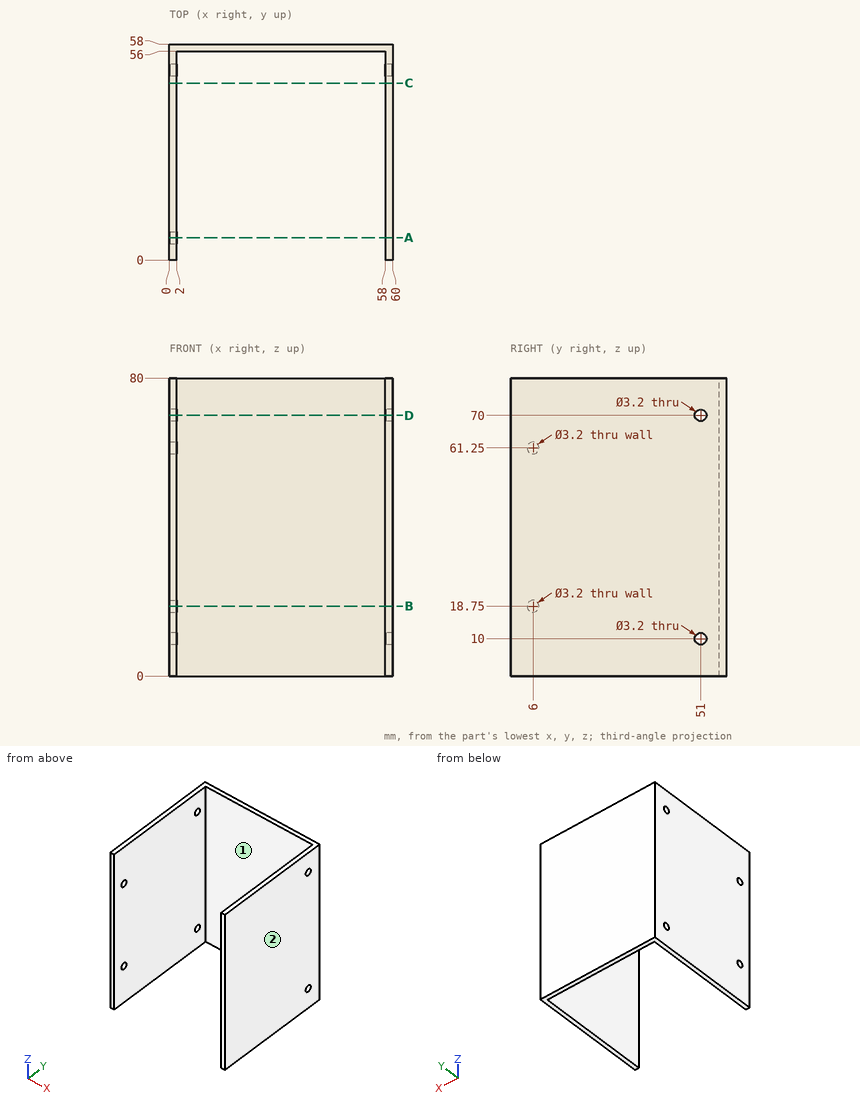
Part print with two shaded views. Sizes in mm from the minimum x, y, z corner. A direction names the side the tool comes from. Round coordinates to 2 decimals unless told otherwise and drop trailing zeros. Write each loop counter-clockwise with the first axis right and the second up, starting at its lowest first coordinate (ties: lowest second). Pieces come first, ordered by that corner, then holes. Notation, with made-up numbers: M 80,34.25 L 116,34.25 A24 ccw 116,58.25 Z; hole C -40,75.25 d4. An arc over 180 degrees is marked long. Answer as CSV lines item,"result". Start each with the question number.
1) Band-saw the part on A-A (y = 6). List the corners of the cut face in (x, z).
2) Band-saw the part on C-C (y = 47.5). List the corners of the cut face in (x, z), then the cut area to 3 significant figures.
3) Band-saw the part on D-D (z = 70). List the corners of the cut face in (x, y), then the cut area to 3 significant figures.
4) Band-saw the part on B-B (z = 18.75). List the corners of the cut face in (x, y).
5) Which spindle directions (+Z, -Z, +X, -X, +Y, -Y) get a long thin tool onto all of the face, cutting with end or side? Do the marked faces 1 and 2. Say none if no direction does.
6) Drill centre lines: L1, parallel to Z at x = 59, y = 51; L2, parallel to X at y = 25.5, z = 7; L3, parallel to Y at x = 0.65, z = 61.25. Where is each one in solid material? Low to high.
7) Drop flat-ended pins along their axis: pin 1 (1.9 mm diameter, centred on y = 51, z = 10, fed in from +X); pin 2 (3 mm diameter, centred on y = 6, z = 18.75, fed in from -X). Give the stop position or say it passes through.
Worked out:
1,outline,"M 0,0 L 2,0 L 2,17.15 L 0,17.15 Z; M 0,20.35 L 2,20.35 L 2,59.65 L 0,59.65 Z; M 0,62.85 L 2,62.85 L 2,80 L 0,80 Z; M 58,0 L 60,0 L 60,80 L 58,80 Z"
2,outline,"M 0,0 L 2,0 L 2,80 L 0,80 Z; M 58,0 L 60,0 L 60,80 L 58,80 Z"
2,area,"320 mm²"
3,outline,"M 0,0 L 2,0 L 2,49.4 L 0,49.4 Z; M 0,52.6 L 2,52.6 L 2,56 L 58,56 L 58,52.6 L 60,52.6 L 60,58 L 0,58 Z; M 58,0 L 60,0 L 60,49.4 L 58,49.4 Z"
3,area,"331 mm²"
4,outline,"M 0,0 L 2,0 L 2,4.4 L 0,4.4 Z; M 0,7.6 L 2,7.6 L 2,56 L 58,56 L 58,0 L 60,0 L 60,58 L 0,58 Z"
5,face 1,"+Z, -Z, -Y"
5,face 2,"+Z, -Z, +X, +Y, -Y"
6,L1,"0 to 8.4, 11.6 to 68.4, 71.6 to 80"
6,L2,"0 to 2, 58 to 60"
6,L3,"0 to 4.4, 7.6 to 58"
7,pin 1,"through"
7,pin 2,"x = 58"
